from build123d import *

# Parameters (mm, degrees)
BOSS_EXTRUDE1_DEPTH = 2.5
CUT_EXTRUDE1_REACH  = 59.935
SKETCH2_R           = 2


with BuildPart() as part:
    # Sketch1 → Boss-Extrude1 (new, symmetric)
    with BuildSketch(Plane(origin=(0, 0, 0), x_dir=(1, 0, 0), z_dir=(0, 1, 0))):
        Polygon((-9.999056518, 49.5), (-14.999056518, 49.5), (-14.999056518, -7), (15.000943482, -7), (15.000943482, 6), (2.115656451, 49.5), (-1.999056518, 49.5), (-1.999056518, 40.504950791), (9.999056518, 0), (-9.999056518, 0), align=None)
    extrude(amount=BOSS_EXTRUDE1_DEPTH, both=True)

    # Cut-Extrude1: up to this face of the body (flat: up to its plane)
    cut_extrude1_end = Plane(part.part.faces().sort_by_distance((15.000943482, 0, 0.5))[0])
    # Sketch2 → Cut-Extrude1 (cut, up to the picked face)
    with BuildSketch(Plane.ZY.offset(14.999056518), mode=Mode.PRIVATE) as cut_extrude1_sk1:
        with Locations(Location((-46.5, 0, 0), (0, 0, 180))):
            Circle(SKETCH2_R)
    cut_extrude1_tool1 = split(extrude(cut_extrude1_sk1.sketch, amount=-CUT_EXTRUDE1_REACH, mode=Mode.PRIVATE), bisect_by=cut_extrude1_end, keep=Keep.BOTH, mode=Mode.PRIVATE)
    # Sketch2 → Cut-Extrude1 (cut, up to the picked face)
    with BuildSketch(Plane.ZY.offset(14.999056518), mode=Mode.PRIVATE) as cut_extrude1_sk2:
        with Locations(Location((-28, 0, 0), (0, 0, 180))):
            Circle(SKETCH2_R)
    cut_extrude1_tool2 = split(extrude(cut_extrude1_sk2.sketch, amount=-CUT_EXTRUDE1_REACH, mode=Mode.PRIVATE), bisect_by=cut_extrude1_end, keep=Keep.BOTH, mode=Mode.PRIVATE)
    # Sketch2 → Cut-Extrude1 (cut, up to the picked face)
    with BuildSketch(Plane.ZY.offset(14.999056518), mode=Mode.PRIVATE) as cut_extrude1_sk3:
        with Locations((3.5, 0)):
            Circle(SKETCH2_R)
    cut_extrude1_tool3 = split(extrude(cut_extrude1_sk3.sketch, amount=-CUT_EXTRUDE1_REACH, mode=Mode.PRIVATE), bisect_by=cut_extrude1_end, keep=Keep.BOTH, mode=Mode.PRIVATE)
    add(cut_extrude1_tool1.solids().sort_by(Axis((-14.999057, 0, -46.5), (1, 0, 0)))[0], mode=Mode.SUBTRACT)
    add(cut_extrude1_tool2.solids().sort_by(Axis((-14.999057, 0, -28), (1, 0, 0)))[0], mode=Mode.SUBTRACT)
    add(cut_extrude1_tool3.solids().sort_by(Axis((-14.999057, 0, 3.5), (1, 0, 0)))[0], mode=Mode.SUBTRACT)


solid = part.part
Design review of the part built by this model. Coordinates are the model's own, in mm. A direction names the side the tool comes from. Coordinates: 2 decimals unless noted, no trailing zeros. Write each loop counter-clockwise with the first axis right and the second up, starting at its lowest first coordinate (ties: lowest second). Pieces come first, ordered by that corner, then holes. Notation, with made-up numbers: (-35.5, 0) - (0.5, 0) arc R16 cw to (0.5, 16) - close; hole circle Ø5 at (56, -0.75). An arc over 180 degrees is marked (long way). Use one line per item in the form item = value.
Q1. Consider section B-B (y = 0.95). Count the separate pieces of the cut face and the enclosed holes in it, plus the area to 3 significant figures.
Taken from the geometry:
separate_pieces = 6
enclosed_holes = 0
area = 593 mm^2
Q2. Consider section C-C (x = 0.5). Write out the cut boundary in (y, z).
Taken from the geometry:
outline = (-2.5, -49.5) - (2.5, -49.5) - (2.5, -32.07) - (-2.5, -32.07) - close; (-2.5, 0) - (2.5, 0) - (2.5, 7) - (-2.5, 7) - close; hole circle Ø4 at (0, -46.5); hole circle Ø4 at (0, 3.5)
Q3. Consider section A-A (z = 3.5). Write out the cut boundary in (x, y).
Taken from the geometry:
outline = (-15, -2.5) - (15, -2.5) - (15, -2) - (-15, -2) - close; (-15, 2) - (15, 2) - (15, 2.5) - (-15, 2.5) - close
Q4. For probe 1 along Y at (x, z) = (-11.25, -46.5); probe 2 along Z at (x, y) = (-11.5, -0.95); probe 3 along X at (y, z) = (0.85, -19), list the stretches that pass through material, from the lowest coordinate up.
Taken from the geometry:
probe_1 = -2.5 to -2, 2 to 2.5
probe_2 = -49.5 to -48.26, -44.74 to -29.76, -26.24 to 1.74, 5.26 to 7
probe_3 = -15 to -10, 4.37 to 11.15
Q5. Machinability: for faces 1 (the flat face through (-9.999, 0, -24)), 2 (the cylindrical face through (-12.534, -0.088, -44.502)), 3 (the flat face through (3.916, 0.035, -20.536)), which of the approach directions +Z, -Z, +X, -X, +Y, -Y give a long, thin tool a straight path to every point of the face, cutting with its end or side? Answer none if there is none.
Taken from the geometry:
face_1 = -Z, +Y, -Y
face_2 = +X, -X
face_3 = +Y, -Y
Q6. The part is to be moulded in two halves that separate along X. For faces 4 (the flat face through (0, 0, 0)), 5 (the flat face through (-1.999, 0, -44)), 6 (the flat face through (10.08, 0.04, -22.61)), 7 (the cylindrical face through (-12.534, -0.601, -29.908)), say which applies: +X half, -X half, draft (parallel to the pull), parting line (faces both ways), or undercut.
Taken from the geometry:
face_4 = undercut
face_5 = undercut
face_6 = +X half
face_7 = draft
Q7. Insertion check: pin 1 Ø6 at (x, z) = (-5.5, -10) entering from -Y; pin 2 Ø1 at (x, y) = (-6, -1.5) entering from -Z; pin 3 Ø1 at (y, z) = (1, -37.5) entering from +X. Each pin has a flat end and moves straight along its axis. Give the tip position at first contact, or say it passes through.
Taken from the geometry:
pin_1 = through
pin_2 = 0
pin_3 = 5.82
Q8. Consider section D-D (z = -46.5). Write out the cut boundary in (x, y), plus the area to 3 significant figures.
Taken from the geometry:
outline = (-15, -2.5) - (-10, -2.5) - (-10, -2) - (-15, -2) - close; (-15, 2) - (-10, 2) - (-10, 2.5) - (-15, 2.5) - close; (-2, -2.5) - (3, -2.5) - (3, -2) - (-2, -2) - close; (-2, 2) - (3, 2) - (3, 2.5) - (-2, 2.5) - close
area = 10.0 mm^2
